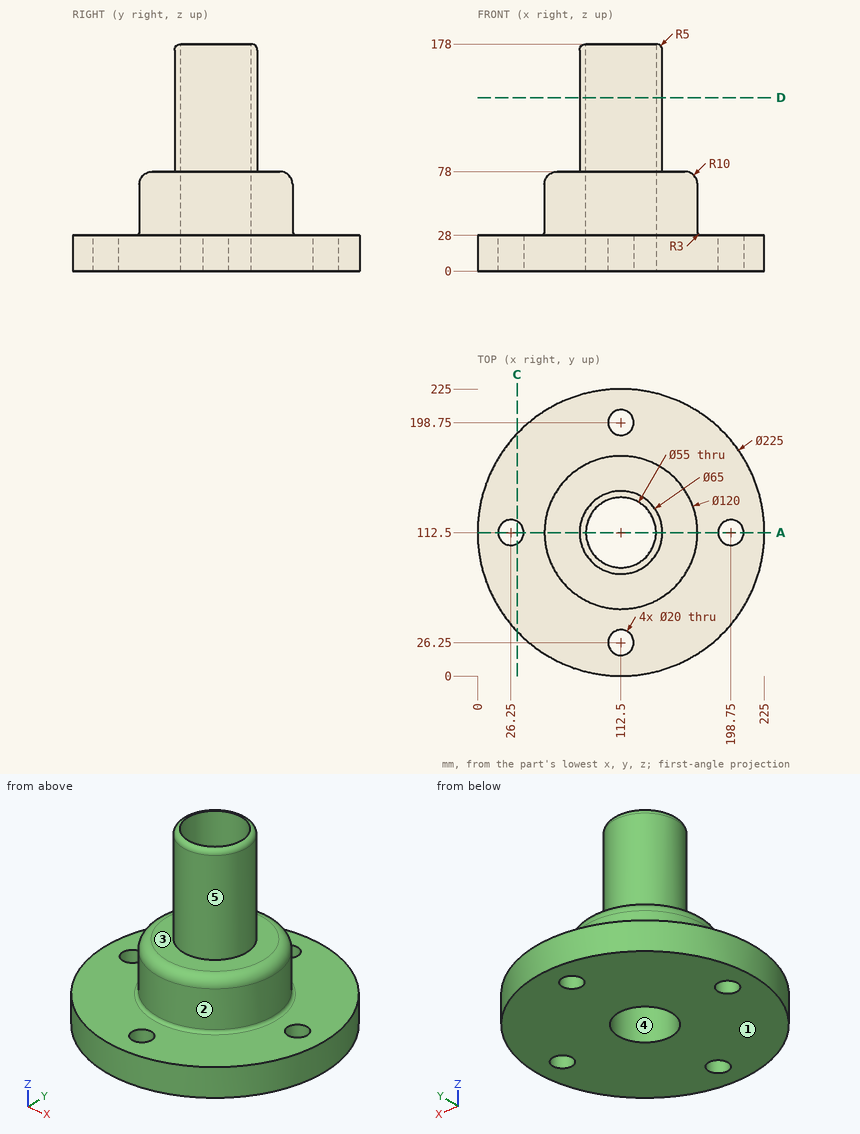
Drawing for the job (mm, zero at the part's lowest x, y, z). A direction names the side the tool comes from. Give positions to 0.01 mm unless a question says otherwise; leave off trailing zeros. Order: outer loops, then holes, each group sorted by start corner. A loop starts at its lowest first (then second) coordinate and runs counter-clockwise, first axis right, second up. Notation, with made-up numbers: M 69,-6.75 L 112,-6.75 A32 cw 112,21.25 Z; hole C 81.5,50.5 d5. An arc over 180 degrees is marked long. Put each result on its own line as item: value. Start each with the question number.
(1) Flat gauge pins, fed straight in: pin 1 Ø5 at (y, z) = (114, 157) entering from +X; pin 2 Ø1.5 at (y, z) = (85, 18.5) entering from +X; pin 3 Ø6 at (x, z) = (64.5, 73) entering from +Y. Where does each tip first touch, or does it go through?
(2) Which spindle directions (+Z, -Z, +X, -X, +Y, -Y) get a long thin tool onto all of the face, cutting with end or side? Do the marked faces 1 and 2. Say none if no direction does.
(3) Drill centre lines: line 1 along Y through (x, z) = (112.5, 11); line 2 along Y through (x, z) = (112, 103); line 3 along Z through (x, y) = (198.5, 139.5). Where is each one in solid material? Low to high.
(4) Saw through at C-C, the plane x = 31. Write the cut outline in (y, z).
(5) Saw through at D-D, the plane z = 136. Write the cut outline in (x, y).
(6) Mould opens along X. For the marked faces 3, 4 and 5 say: +X half, -X half, draft (parallel to the pull), parting line (faces both ways), or undercut.
(7) Saw through at A-A, the plane y = 112.5. Give the number of separate pieces and of enclosed holes in the cut face, then the cut area to 3 significant figures.
Check result:
1. pin 1: stops at x = 145
1. pin 2: stops at x = 221.77
1. pin 3: stops at y = 150.76
2. face 1: -Z, +X, -X, +Y, -Y
2. face 2: +Z
3. line 1: y = 0 to 16.25, 36.25 to 85, 140 to 188.75, 208.75 to 225
3. line 2: y = 80 to 85, 140 to 145
3. line 3: z = 0 to 28
4. outline: M 34.95,0 L 103.7,0 L 103.7,28 L 34.95,28 Z; M 121.3,0 L 190.05,0 L 190.05,28 L 121.3,28 Z
5. outline: C 112.5,112.5 d65; hole C 112.5,112.5 d55
6. face 3: draft
6. face 4: undercut
6. face 5: parting line
7. separate pieces: 4
7. enclosed holes: 0
7. area: 7,840 mm2
